Input: part model. Units: mm. Frame: model coordinates. Face numbers are marked on the shaded views. Coordinates: 2 decimals unless noted, no trailing zeros. Loops run counter-clockwise (first coordinate to the right, second up) from the corner with the lowest first, then second, coordinate; pieces in that order, holes last. Notation, with made-up numbers: (51.25, 54.5) -> (65.25, 54.5) arc R20 ccw to (65.25, 79.5) -> close; hole circle Ø5 at (-29.75, -28). An arc over 180 degrees is marked (long way). Put each result on its own line as item: value. Start each with the question number.
1) Material intervals for L1, parallel to Y at x = 16.5, z = 168.5; L2, parallel to Y at x = 7.75, z = 170; L3, parallel to Z at x = 9, y = 4, sorted ascending.
2) Contact query for flat-ended pins moving along their axis: P1, Ø5, axis at x = 9, z = 27, coming from the +Y side; P2, Ø1.5, axis at x = 13.5, y = 22.5, coming from the +Z side; P3, Ø1.5, axis at x = 16, y = 83, coming from the +Z side; P4, Ø2.5, axis at x = 9, z = 112, coming from the -Y side. Output: stop coordinate, or through.
3) Pull-direction query (X, two-part tool) for the marked faces 1 and 2; classes: pulls with the +X half, pulls with the -X half, needs draft (parallel to the pull), parting line crosses it, or undercut.
4) Cut plane B-B (y = 82.5). Return the cut outline in (x, z).
5) Cut plane A-A (z = 170). Return the cut outline in (x, y), plus the area to 3 significant figures.
6) Cut plane C-C (y = 37.5). Return the cut outline in (x, z).
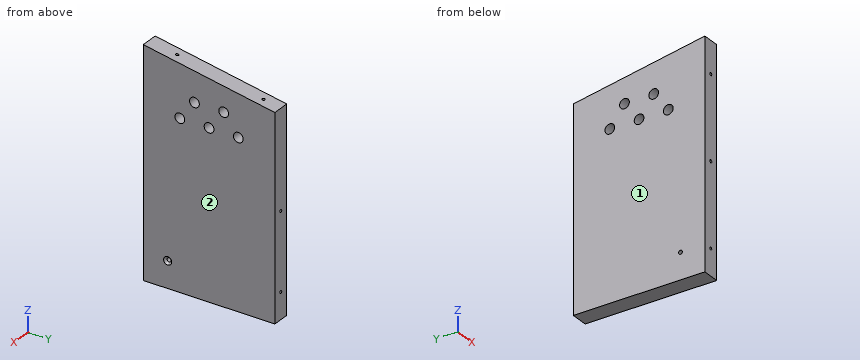
from build123d import *

# Parameters (mm, degrees)
F1_DEPTH       = 18
F2_D           = 10
F3_D           = 10
F5_D           = 4
F5_CSINK_D     = 8.2
F5_CSINK_ANGLE = 90
F7_D           = 3
F7_DEPTH       = 20
F7_TIP         = 0.9012909285
F9_D           = 3
F9_DEPTH       = 20
F9_TIP         = 0.9012909285
F11_D          = 3
F11_DEPTH      = 20
F11_TIP        = 0.9012909285


# Not quite as in the source:
# - a feature names something its author has since deleted; it is built from what else it names


with BuildPart() as f1:
    # F0 (on Right) → F1 (new body)
    with BuildSketch(Plane.YZ):
        Polygon((0, 230), (0, 0), (135, 0), (135, 206.1958576044), align=None)
    extrude(amount=F1_DEPTH)

    # F2 (through all)
    with Locations(Plane(origin=(0, 0, 0), x_dir=(0, 1, 0), z_dir=(-1, 0, 0))):
        with Locations((37.5, -170), (67.5, -170), (97.5, -170)):
            Hole(F2_D / 2)

    # F3 (through all)
    with Locations(Plane(origin=(0, 0, 0), x_dir=(0, 1, 0), z_dir=(-1, 0, 0))):
        with Locations((52.5, -190), (82.5, -190)):
            Hole(F3_D / 2)

    # F5 (through all)
    with Locations(Plane.YZ.offset(18)):
        with Locations((25, 27)):
            CounterSinkHole(F5_D / 2, F5_CSINK_D / 2, counter_sink_angle=F5_CSINK_ANGLE)

    # F7
    with Locations(Plane(origin=(0, 135, 0), x_dir=(-1, 0, 0), z_dir=(0, 1, 0))):
        with Locations((-9, 27), (-9, 106)):
            Hole(F7_D / 2, depth=F7_DEPTH)
            with Locations((0, 0, -(F7_DEPTH + F7_TIP / 2))):  # 118° drill point
                Cone(0, F7_D / 2, F7_TIP, mode=Mode.SUBTRACT)

    # F9
    with Locations(Plane.XZ):
        with Locations((9, 197), (9, 112), (9, 27)):
            Hole(F9_D / 2, depth=F9_DEPTH)
            with Locations((0, 0, -(F9_DEPTH + F9_TIP / 2))):  # 118° drill point
                Cone(0, F9_D / 2, F9_TIP, mode=Mode.SUBTRACT)

    # F11
    with Locations(Plane(origin=(0, 39.3323164825, 223.0646513904), x_dir=(1, 0, 0), z_dir=(0, 0.1736481777, 0.984807753))):
        with Locations((9, -10.8564882588), (9, 79.1435117412)):
            Hole(F11_D / 2, depth=F11_DEPTH)
            with Locations((0, 0, -(F11_DEPTH + F11_TIP / 2))):  # 118° drill point
                Cone(0, F11_D / 2, F11_TIP, mode=Mode.SUBTRACT)


solid = f1.part
Results found:
1. L1: y = 0 to 32.73, 42.27 to 62.73, 72.27 to 92.73, 102.27 to 135
1. L2: y = 0 to 32.5, 42.5 to 62.5, 72.5 to 92.5, 102.5 to 135
1. L3: z = 0 to 25.5, 28.5 to 110.5, 113.5 to 195.5, 198.5 to 229.29
2. P1: stops at y = 135
2. P2: stops at z = 226.16
2. P3: stops at z = 215.5
2. P4: stops at y = 20.15
3. face 1: pulls with the -X half
3. face 2: pulls with the +X half
4. outline: (0, 0) -> (18, 0) -> (18, 185) -> (0, 185) -> close; (0, 195) -> (18, 195) -> (18, 215.45) -> (0, 215.45) -> close
5. outline: (0, 0) -> (18, 0) -> (18, 32.5) -> (0, 32.5) -> close; (0, 42.5) -> (18, 42.5) -> (18, 62.5) -> (0, 62.5) -> close; (0, 72.5) -> (18, 72.5) -> (18, 92.5) -> (0, 92.5) -> close; (0, 102.5) -> (18, 102.5) -> (18, 135) -> (0, 135) -> close
5. area: 1,890 mm2
6. outline: (0, 0) -> (18, 0) -> (18, 165) -> (0, 165) -> close; (0, 175) -> (18, 175) -> (18, 223.39) -> (0, 223.39) -> close
